For this review, take the finished solid that the model builds, in its own axes (mm). Face numbers are marked on the shaded views. Give positions to 0.01 mm unless a question says otherwise; leave off trailing zeros. Write each loop counter-clockwise with the first axis right and the second up, starting at its lowest first coordinate (ties: lowest second). Pieces come first, ordered by that corner, then holes. Notation, with made-up numbers: M 64.5,32.25 L 91.5,32.25 A24 ccw 91.5,55.25 Z; hole C -22.5,-28 d2. An arc over 180 degrees is marked long. Use one line per item in the form item = value. Start each with the question number.
Q1. Consider section B-B on z = -35. Write out the cut boundary in (x, y).
Q2. Clearance check with flat-ended pins moving along their axes: pin 1 Ø5 at (x, y) = (-175, 4) entering from -Z; pin 2 Ø2 at (x, y) = (-185, -2.5) entering from +Z; pin 3 Ø1 at (x, z) = (-178, -30.5) entering from +Y; pin 4 Ø12 at (y, z) = (0, -37.45) entering from -X. State where each tip first meets the part, or that it passes through.
Q3. Mouldability with a two-part tool opening along Z and no side actions: class the marked faces 1, 2, 3 and 4 as released by +Z, released by -Z, zero draft, split by the parting line, or undercut.
Q4. For probe 1 along Y at (x, z) = (-165, -28.5); probe 2 along Z at (x, y) = (-179.5, 0); probe 3 along Y at (x, z) = (-165.75, -38), list the stretches that pass through material, from the lowest coordinate up. Write a range as [from, to].
Q5. Consider section A-A on y = 3.25. Write out the cut boundary in (x, z), and give its area (3 significant figures).
```python
from build123d import *

# Parameters (mm, degrees)
F0_W     = 28.3845
F0_H     = 3.72745
F3_DEPTH = 28.3855
F4_COUNT = 12


with BuildPart() as f1:
    # F0 (on Front) → F1 (revolve)
    with BuildSketch(Plane.XZ):
        with Locations((-177.8664920464, -27.9698891753)):
            Rectangle(F0_W, F0_H)
    revolve(axis=Axis((-177.8664920464, 0, -37.4536141753), (1, 0, 0)))

    # F2 (on face) → F3 (cut, through all)
    with BuildSketch(Plane(origin=(-192.0587420464, 0, 0), x_dir=(0, -1, 0), z_dir=(-1, 0, 0))):
        with BuildLine():
            Line((1.39065, -26.4860777063), (1.39065, -26.1916998585))
            ThreePointArc((1.39065, -26.1916998585), (0, -26.1061641753), (-1.39065, -26.1916998585))
            Line((-1.39065, -26.1916998585), (-1.39065, -26.4860777063))
            ThreePointArc((-1.39065, -26.4860777063), (0, -26.3982641753), (1.39065, -26.4860777063))
        make_face()
    f3 = extrude(amount=-F3_DEPTH, mode=Mode.SUBTRACT)

    # F4: F3 ×12 about axis
    f4_axis = Axis((-163.6742420464, 0, -37.4536141753), (-1, 0, 0))
    for i in range(1, F4_COUNT):
        add(f3.rotate(f4_axis, i * 360 / F4_COUNT), mode=Mode.SUBTRACT)


solid = f1.part
```
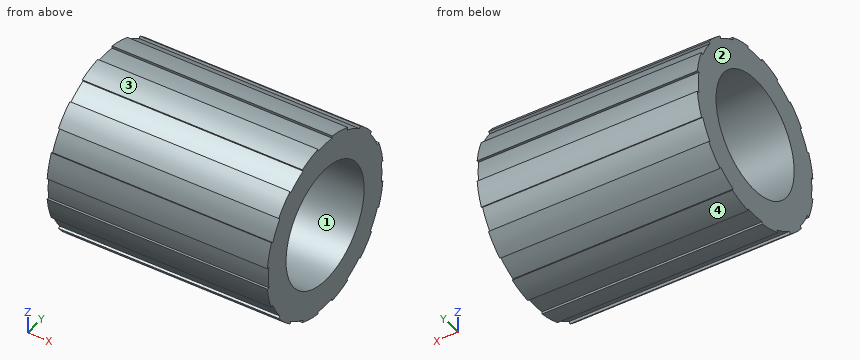
Working result:
q1.outline = M -192.06,-11.08 L -163.67,-11.08 L -163.67,-7.21 L -192.06,-7.21 Z; M -192.06,7.21 L -163.67,7.21 L -163.67,11.08 L -192.06,11.08 Z
q2.pin_1 = -48.7
q2.pin_2 = -26.21
q2.pin_3 = 9.06
q2.pin_4 = through
q3.face_1 = undercut
q3.face_2 = zero draft
q3.face_3 = released by +Z
q3.face_4 = released by -Z
q4.probe_1 = [-6.97, -6.78], [-6.48, 6.48], [6.78, 6.97]
q4.probe_2 = [-48.51, -45.07], [-29.83, -26.4]
q4.probe_3 = [-11.04, -7.6], [7.6, 11.04]
q5.outline = M -192.06,-48.33 L -163.67,-48.33 L -163.67,-44.35 L -192.06,-44.35 Z; M -192.06,-30.56 L -163.67,-30.56 L -163.67,-26.58 L -192.06,-26.58 Z
q5.area = 226 mm²
